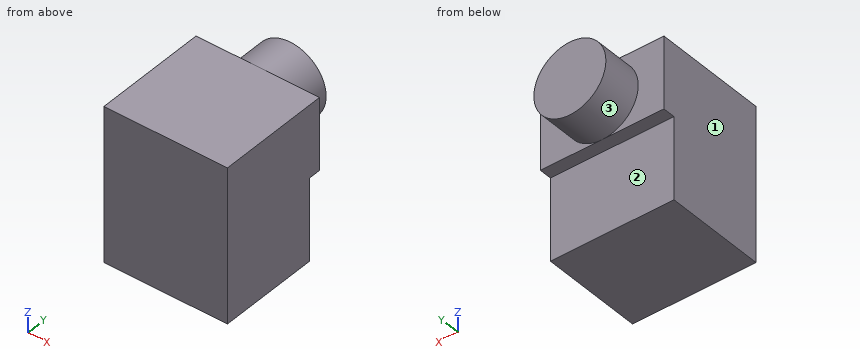
Autodesk Inventor part; units mm, degrees
ref_plane "YZ Plane" through (0, 0, 0) normal (1, 0, 0) x (0, 1, 0)
ref_plane "XZ Plane" through (0, 0, 0) normal (0, 1, 0) x (-1, 0, 0)
ref_plane "XY Plane" through (0, 0, 0) normal (0, 0, 1) x (1, 0, 0)
sketch "Sketch1" plane through (0, 0, 0) normal (0, 1, 0) x (-1, 0, 0)
  line L0 (0, 0) -> (12.0142, 0)
  line L1 (12.0142, 0) -> (12.0142, -7.0104)
  line L2 (12.0142, -7.0104) -> (0, -7.0104)
  line L3 (0, -7.0104) -> (0, 0)
  circle A0 centre (6.0071, -3.5052) radius 3.5052
  line L4 (12.0142, 0) -> (0, 0)
  line L5 (0, 0) -> (0, -15.0114)
  line L6 (0, -15.0114) -> (12.0142, -15.0114)
  line L7 (12.0142, -15.0114) -> (12.0142, 0)
  point P0 (0, -3.5052)
  point P1 (6.0071, -7.0104)
  point P2 (6.0071, 0)
  dimension "d0" = 12.0142
  dimension "d1" = 7.0104
  dimension "d2" = 3.5052
  dimension "d3" = 6.0071
  dimension "d4" = 7.0104
  dimension "d5" = 15.0114
extrude "Extrusion1" add sketch "Sketch1" along normal blind 9.906 contours L2 L7 L6 L5
extrude "Extrusion2" add sketch "Sketch1" along normal blind 11.1125 contours L0 A0 L2 L3 | L0 L1 L2 A0
extrude "Extrusion3" add sketch "Sketch1" along normal blind 15.0114 contours A0
properties part number "Audio_jack"
Source: CAD feature listing. Evaluate the final solid. Frame: model axes, mm. Face numbers are marked on the shaded views. A direction names the side the tool comes from. Give positions to 0.01 mm unless a question says otherwise; leave off trailing zeros. Write each loop counter-clockwise with the first axis right and the second up, starting at its lowest first coordinate (ties: lowest second). Pieces come first, ordered by that corner, then holes. Notation, with made-up numbers: M 2.5,85.25 L 16.5,85.25 A14 cw 16.5,102.25 Z; hole C -8.5,75.25 d11. An arc over 180 degrees is marked long. Return JSON: item names as keys, results as strings. Group by question number.
1) Material intervals for line 1 along Y through (x, z) = (-2, -14); line 2 along Y through (x, z) = (-10.25, -6.75); line 3 along X through (y, z) = (13.5, -5), sorted ascending. Write a range as [from, to].
2) Pin query (flat end, axial travel): P1, Ø4, axis at x = -6.5, z = -9.5, coming from the +Y side. Return the tip coordinate at first contact, or that it passes through.
3) Set-up query: the marked faces 1, 2 and 3. Return all of +Z, -Z, +X, -X, +Y, -Y with unobstructed straight access to the full face (end or side cutting, diameter ignored); none if empty.
4) Cut plane C-C, the plane z = -6. Output: boundary loops of the cut face in (x, y), plus the area to 3 significant figures.
5) Cut plane D-D, the plane x = -9.75. Output: boundary loops of the cut face in (y, z), plus the area to 3 significant figures.
6) Cut plane B-B, the plane z = -11.25. Output: boundary loops of the cut face in (x, y).
7) Cut plane A-A, the plane x = -4. Output: boundary loops of the cut face in (y, z).
Recorded:
{
 "1": {"line 1": "y = [0, 9.91]", "line 2": "y = [0, 11.11]", "line 3": "x = [-9.18, -2.84]"},
 "2": {"P1": "stops at y = 9.91"},
 "3": {"face 1": "+Z, -Z, -X, +Y, -Y", "face 2": "-Z, +X, -X, +Y", "face 3": "+Y"},
 "4": {"outline": "M -12.01,0 L 0,0 L 0,11.11 L -3.54,11.11 L -3.54,15.01 L -8.47,15.01 L -8.47,11.11 L -12.01,11.11 Z", "area": "153 mm²"},
 "5": {"outline": "M 0,-15.01 L 9.91,-15.01 L 9.91,-7.01 L 11.11,-7.01 L 11.11,0 L 0,0 Z", "area": "157 mm²"},
 "6": {"outline": "M -12.01,0 L 0,0 L 0,9.91 L -12.01,9.91 Z"},
 "7": {"outline": "M 0,-15.01 L 9.91,-15.01 L 9.91,-7.01 L 11.11,-7.01 L 11.11,-6.38 L 15.01,-6.38 L 15.01,-0.63 L 11.11,-0.63 L 11.11,0 L 0,0 Z"}
}
